Part model, mm, in its own coordinate system. Round coordinates to 2 decimals unless told otherwise and drop trailing zeros. Order: outer loops, then holes, each group sorted by start corner. A loop starts at its lowest first (then second) coordinate and runs counter-clockwise, first axis right, second up. Notation, with made-up numbers: (67, -23.5) -> (112, -23.5) arc R31 ccw to (112, 12.5) -> close; hole circle Ø7 at (21.25, -27). An arc over 180 degrees is marked (long way). Use CSV: the item, a comma, the result in double quotes.
```python
from build123d import *

# Parameters (mm, degrees)
SKETCH1_W            = 2000
SKETCH1_H            = 1100
BOSS_EXTRUDE1_DEPTH  = 500
SHELL1_T             = 10
SKETCH2_W            = 150
SKETCH2_H            = 200
BOSS_EXTRUDE2_DEPTH  = 200
LPATTERN1_COUNT      = 4
LPATTERN1_PITCH      = 400
LPATTERN1_COUNT_DIR2 = 2
LPATTERN1_PITCH_DIR2 = 350


with BuildPart() as part:
    # Sketch1 → Boss-Extrude1 (new body)
    with BuildSketch(Plane(origin=(0, 0, 0), x_dir=(1, 0, 0), z_dir=(0, 1, 0))):
        with Locations((1000, 550)):
            Rectangle(SKETCH1_W, SKETCH1_H)
    extrude(amount=BOSS_EXTRUDE1_DEPTH)

    # Shell1
    shell1_openings = [part.faces().sort_by_distance(p)[0] for p in [
        (1000, 500, -550),
    ]]
    offset(amount=SHELL1_T, openings=shell1_openings, kind=Kind.INTERSECTION)

    # Sketch2 → Boss-Extrude2 (add)
    with BuildSketch(Plane(origin=(0, 0, 0), x_dir=(1, 0, 0), z_dir=(0, 1, 0))):
        with Locations((375, 400)):
            Rectangle(SKETCH2_W, SKETCH2_H)
    boss_extrude2 = extrude(amount=BOSS_EXTRUDE2_DEPTH)

    # LPattern1: Boss-Extrude2 4 × 2
    with Locations(*[(i * LPATTERN1_PITCH, 0, -j * LPATTERN1_PITCH_DIR2) for i in range(LPATTERN1_COUNT) for j in range(LPATTERN1_COUNT_DIR2) if (i, j) != (0, 0)]):
        add(boss_extrude2)


solid = part.part
```
(1) Probe probe 1 along Z at (x, y) = (380, 101.5); probe 2 along X at (y, z) = (157, -465); probe 3 along Z at (x, y) = (1738, 455). List the from-to ranges inside material, lowest first. Write a range as [from, to].
Reply:
probe 1,"[-1110, -1100], [-850, -650], [-500, -300], [0, 10]"
probe 2,"[-10, 0], [300, 450], [700, 850], [1100, 1250], [1500, 1650], [2000, 2010]"
probe 3,"[-1110, -1100], [0, 10]"
(2) Cut at D-D, the plane y = 64. State how many separate pieces and enclosed holes the cut face has, then the cut area to 3 significant figures.
Reply:
separate pieces,"9"
enclosed holes,"1"
area,"302,000 mm2"
(3) Cut at A-A, the plane y = 248.5. Give the cut face in (x, z), then the cut area to 3 significant figures.
Reply:
outline,"(-10, -1110) -> (2010, -1110) -> (2010, 10) -> (-10, 10) -> close; hole (0, -1100) -> (2000, -1100) -> (2000, 0) -> (0, 0) -> close"
area,"62,400 mm2"
(4) Pull direction X, two halves, no side cores. Call faces 1 (the face through (450, 99, -749)), 2 (the face through (986, -10, -558)): released by +X, released by -X, zero draft, split by the parting line, or undercut.
Reply:
face 1,"undercut"
face 2,"zero draft"
(5) Cut at C-C, the plane x = 763. Give the cut face in (y, z).
Reply:
outline,"(-10, -1110) -> (500, -1110) -> (500, -1100) -> (0, -1100) -> (0, -850) -> (200, -850) -> (200, -650) -> (0, -650) -> (0, -500) -> (200, -500) -> (200, -300) -> (0, -300) -> (0, 0) -> (500, 0) -> (500, 10) -> (-10, 10) -> close"
(6) Cut at B-B, the plane z = -184.5. Give the cut face in (x, y), then the cut area to 3 significant figures.
Reply:
outline,"(-10, -10) -> (2010, -10) -> (2010, 500) -> (2000, 500) -> (2000, 0) -> (0, 0) -> (0, 500) -> (-10, 500) -> close"
area,"30,200 mm2"
